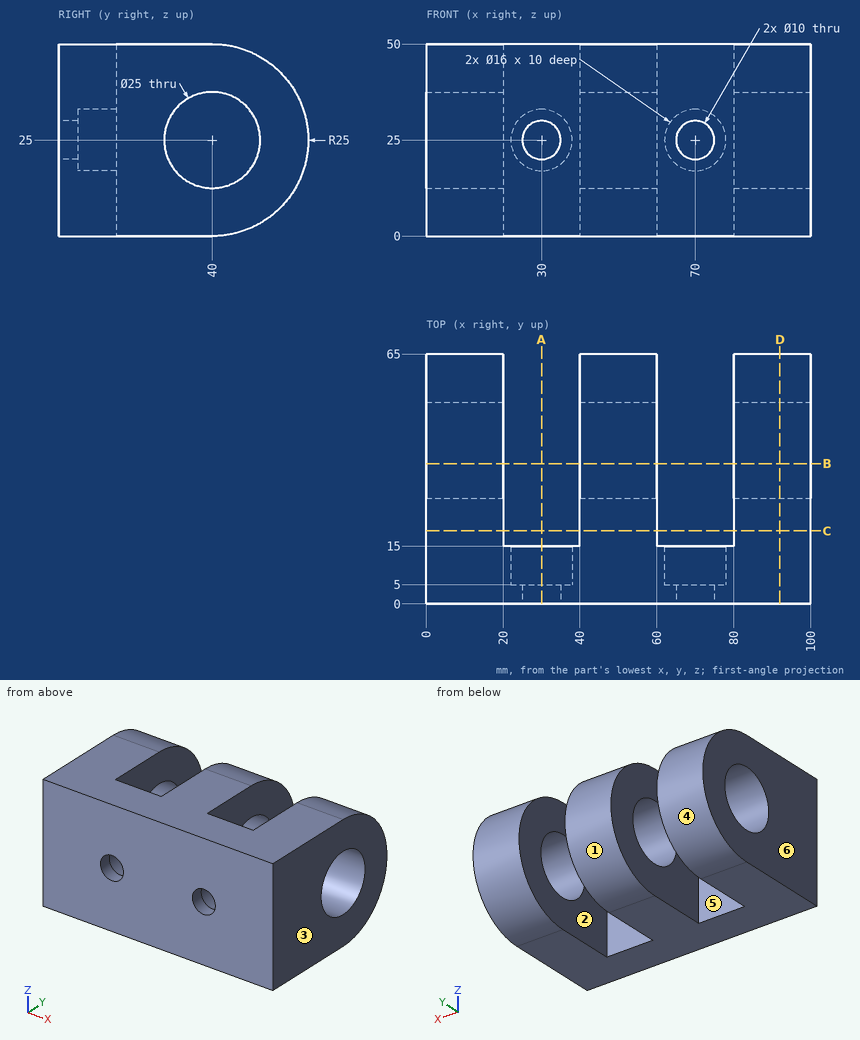
Source: three-view drawing plus pictorial views. Frame: mm from the lowest corner of the part. A direction names the side the tool comes from. Round coordinates to 2 decimals unless told otherwise and drop trailing zeros. Write each loop counter-clockwise with the first axis right and the second up, starting at its lowest first coordinate (ties: lowest second). Pieces come first, ordered by that corner, then holes. Notation, with made-up numbers: M 77.5,-23.5 L 99.5,-23.5 A18 cw 99.5,7.5 Z; hole C -6,82 d9. An arc over 180 degrees is marked long. Write each question's results on one line, items separated by ' | '.
Q1. Line query: line 1 along X through (y, z) = (17.5, 13.5); line 2 along X through (y, z) = (10.5, 25); line 3 along Z through (x, y) = (70, 10). Output: solid intervals per line, ascending.
Results:
line 1: x = 0 to 20, 40 to 60, 80 to 100 | line 2: x = 0 to 22, 38 to 62, 78 to 100 | line 3: z = 0 to 17, 33 to 50
Q2. Section query D-D (x = 92). Return loops of the section in (y, z), and give its area (3 significant figures).
Results:
outline: M 0,0 L 40,0 A25 ccw 40,50 L 0,50 Z; hole C 40,25 d25 | area: 2,490 mm^2
Q3. Access query for the marked faces 1 and 2. Directions: +Z, -Z, +X, -X, +Y, -Y. A direction counts if a zero-diameter tool reaches every point of the face in a straight line with its end or side. Return the directions, or none.
Results:
face 1: +X, -X, +Y | face 2: +Z, -Z, +Y
Q4. Section query A-A (x = 30). Return loops of the section in (y, z), and give its area (3 significant figures).
Results:
outline: M 0,0 L 15,0 L 15,17 L 5,17 L 5,20 L 0,20 Z; M 0,30 L 5,30 L 5,33 L 15,33 L 15,50 L 0,50 Z | area: 540 mm^2
Q5. Draft query along X for the marked faces 3, 4, 5 and 6. Return one class per face: released by +X, released by -X, zero draft, split by the parting line, or undercut.
Results:
face 3: released by +X | face 4: zero draft | face 5: undercut | face 6: released by -X
Q6. Section query B-B (y = 36.5). Return loops of the section in (x, z).
Results:
outline: M 0,0 L 20,0 L 20,13 L 0,13 Z; M 0,37 L 20,37 L 20,50 L 0,50 Z; M 40,0 L 60,0 L 60,13 L 40,13 Z; M 40,37 L 60,37 L 60,50 L 40,50 Z; M 80,0 L 100,0 L 100,13 L 80,13 Z; M 80,37 L 100,37 L 100,50 L 80,50 Z
Q7. Section query C-C (y = 19). Return loops of the section in (x, z), and give its area (3 significant figures).
Results:
outline: M 0,0 L 20,0 L 20,50 L 0,50 Z; M 40,0 L 60,0 L 60,50 L 40,50 Z; M 80,0 L 100,0 L 100,50 L 80,50 Z | area: 3,000 mm^2
Q8. Pin query (flat end, axial travel): P1, Ø6, axis at x = 90, y = 31, coming from the -Z side; P2, Ø5, axis at x = 81.5, z = 29, coming from the +Y side; P3, Ø17.5, axis at x = 70.5, z = 27.5, coming from the +Y side; P4, Ø3, axis at x = 85, y = 50, coming from the +Z side. Return the tip coordinate at first contact, or that it passes through.
Results:
P1: stops at z = 0 | P2: stops at y = 64.95 | P3: stops at y = 15 | P4: stops at z = 48.51
